```python
from build123d import *

# Parameters (mm, degrees)
ESQUISSE1_R              = 8
ESQUISSE1_R_2            = 1.1
DISQUE_O16_DEPTH         = 1.5
ESQUISSE2_R              = 3.5
ESQUISSE2_R_2            = 2.35
MOYEU_CANNELE_SG90_DEPTH = 3


with BuildPart() as part:
    # Esquisse1 → Disque O16 (new body)
    with BuildSketch(Plane.XY):
        Circle(ESQUISSE1_R)
        with Locations((3.889087297, 3.889087297)):
            Circle(ESQUISSE1_R_2, mode=Mode.SUBTRACT)
        with Locations((-3.889087297, 3.889087297)):
            Circle(ESQUISSE1_R_2, mode=Mode.SUBTRACT)
    extrude(amount=DISQUE_O16_DEPTH)

    # Esquisse2 → Moyeu cannele SG90 (add)
    with BuildSketch(Plane.XY):
        Circle(ESQUISSE2_R)
        Circle(ESQUISSE2_R_2, mode=Mode.SUBTRACT)
    extrude(amount=-MOYEU_CANNELE_SG90_DEPTH)


solid = part.part
```
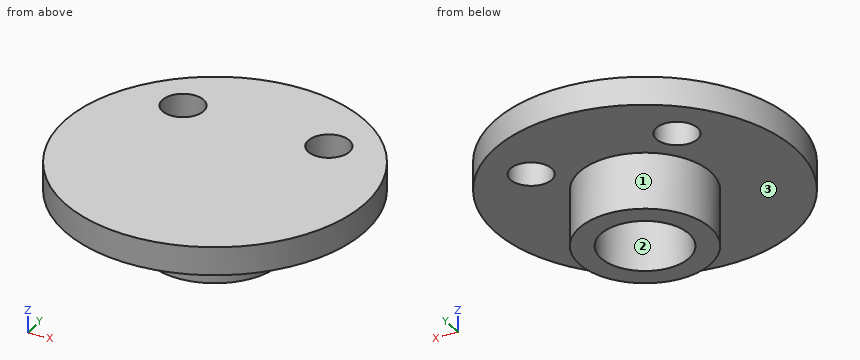
Could you check a few things on this model? Use its own coordinates, in mm. Face numbers are marked on the shaded views. Round coordinates to 2 decimals unless told otherwise and drop trailing zeros. Loops run counter-clockwise (first coordinate to the right, second up) from the corner with the lowest first, then second, coordinate; pieces in that order, holes last. Notation, with made-up numbers: (-39.75, -16.5) - (-5.75, -16.5) arc R20 cw to (-5.75, 8.5) - close; hole circle Ø5 at (-18.5, 37). An arc over 180 degrees is marked (long way). Use CSV: the item, a comma, the result in double quotes.
Item 1: If we section it at A-A on y = 0: List the corners of the cut face in (x, z) for me.
Here are the results:
outline,"(-8, 0) - (-3.5, 0) - (-3.5, -3) - (-2.35, -3) - (-2.35, 0) - (2.35, 0) - (2.35, -3) - (3.5, -3) - (3.5, 0) - (8, 0) - (8, 1.5) - (-8, 1.5) - close"
Item 2: I need wall thicknesses on L1, parallel to Y at x = 0, z = -1.6; L2, parallel to Z at x = 3, y = 2; L3, parallel to Y at x = -1, z = -1.65. Which ranges of each line are inside material? Lowest first, please. Write a range as [from, to].
Here are the results:
L1,"y = [-3.5, -2.35], [2.35, 3.5]"
L2,"z = [0, 1.5]"
L3,"y = [-3.35, -2.13], [2.13, 3.35]"
Item 3: If we section it at C-C on z = -1.65: List the corners of the cut face in (x, y) for me, then the cut area to 3 significant figures.
Here are the results:
outline,"circle Ø7 at (0, 0); hole circle Ø4.7 at (0, 0)"
area,"21.1 mm²"
Item 4: If we section it at D-D on z = 1: List the corners of the cut face in (x, y) for me.
Here are the results:
outline,"circle Ø16 at (0, 0); hole circle Ø2.2 at (-3.89, 3.89); hole circle Ø2.2 at (3.89, 3.89)"
Item 5: Will these pins go through, and if not, where does the flat tip stop? pin 1 (1.5 mm diameter, centred on y = 3.5, z = 0.5, fed in from -X); pin 2 (3 mm diameter, centred on x = 3.89, y = 3.89, fed in from -Z); pin 3 (1.5 mm diameter, centred on y = -2, z = 0, fed in from +X).
Here are the results:
pin 1,"stops at x = -7.51"
pin 2,"stops at z = 0"
pin 3,"stops at x = 7.9"
Item 6: If we mould it in two halves opening along X, with no side actions, what happens to the marked faces 1, 2 and 3? For each: pulls with the +X half, pulls with the -X half, needs draft (parallel to the pull), parting line crosses it, or undercut.
Here are the results:
face 1,"parting line crosses it"
face 2,"undercut"
face 3,"needs draft"
